from build123d import *

# Parameters (mm, degrees)
SKETCH_1_W          = 290
SKETCH_1_H          = 50
EXTRUDE_1_DEPTH     = 5
SKETCH_3_W          = 20
SKETCH_3_H          = 50
CUT_EXTRUDE_1_DEPTH = 10
SKETCH_4_W          = 150
SKETCH_4_H          = 5
EXTRUDE_2_DEPTH     = 10
SKETCH_5_R          = 2.75
CUT_EXTRUDE_4_DEPTH = 130.903810568
CUT_EXTRUDE_5_DEPTH = 10


with BuildPart() as part:
    # 스케치1 → 보스-돌출1 (new body)
    with BuildSketch(Plane.XY):
        Rectangle(SKETCH_1_W, SKETCH_1_H)
    extrude(amount=EXTRUDE_1_DEPTH)

    # 스케치3 → 컷-돌출1 (cut)
    with BuildSketch(Plane.XY.offset(5)):
        with Locations((-135, 0)):
            Rectangle(SKETCH_3_W, SKETCH_3_H)
    cut_extrude_1 = extrude(amount=-CUT_EXTRUDE_1_DEPTH, mode=Mode.SUBTRACT)

    # 대칭 복사1: 컷-돌출1 across plane
    add(cut_extrude_1.mirror(Plane(origin=(0, 0, 0), x_dir=(0, 0, 1), z_dir=(1, 0, 0))), mode=Mode.SUBTRACT)

    # 스케치4 → 보스-돌출2 (add)
    with BuildSketch(Plane(origin=(0, 25, 0), x_dir=(1, 0, 0), z_dir=(0, 1, 0))):
        with Locations((0, -2.5)):
            Rectangle(SKETCH_4_W, SKETCH_4_H)
    extrude(amount=EXTRUDE_2_DEPTH)

    # 스케치5 → 컷-돌출4 (cut, through all)
    with BuildSketch(Plane.XY.offset(5)):
        with Locations((-84, 15)):
            Circle(SKETCH_5_R)
        with Locations((-116, 15)):
            Circle(SKETCH_5_R)
        with Locations(Location((116, 15, 0), (0, 0, 180))):
            Circle(SKETCH_5_R)
        with Locations(Location((84, 15, 0), (0, 0, 180))):
            Circle(SKETCH_5_R)
    extrude(amount=-CUT_EXTRUDE_4_DEPTH, mode=Mode.SUBTRACT)

    # 스케치6 → 컷-돌출5 (cut)
    with BuildSketch(Plane.XY.offset(5)):
        with BuildLine():
            Line((59.99900565, 22.696938457), (59.99900565, -6.696938457))
            ThreePointArc((59.99900565, -6.696938457), (44.99900565, -13), (29.99900565, -6.696938457))
            Line((29.99900565, -6.696938457), (29.99900565, 22.696938457))
            ThreePointArc((29.99900565, 22.696938457), (44.99900565, 29), (59.99900565, 22.696938457))
        make_face()
    cut_extrude_5 = extrude(amount=-CUT_EXTRUDE_5_DEPTH, mode=Mode.SUBTRACT)

    # 대칭 복사2: 컷-돌출5 across plane
    add(cut_extrude_5.mirror(Plane.ZY), mode=Mode.SUBTRACT)


solid = part.part
Work out the finished part from the listing and answer in its coordinate system (mm). A direction names the side the tool comes from. Give positions to 0.01 mm unless a question says otherwise; leave off trailing zeros. Loops run counter-clockwise (first coordinate to the right, second up) from the corner with the lowest first, then second, coordinate; pieces in that order, holes last. Notation, with made-up numbers: (13, 76.5) - (63, 76.5) arc R33 cw to (63, 115.5) - close; hole circle Ø5 at (72, 9). An arc over 180 degrees is marked (long way). Answer in a Markdown table with one row per item.
(1) Section C-C (y = 15) is taken. Give the vertices of the cut face in (x, z), and give its area (3 significant figures).
Results list:
| item | result |
|---|---|
| outline | (-125, 0) - (-118.75, 0) - (-118.75, 5) - (-125, 5) - close; (-113.25, 0) - (-86.75, 0) - (-86.75, 5) - (-113.25, 5) - close; (-81.25, 0) - (-60, 0) - (-60, 5) - (-81.25, 5) - close; (-30, 0) - (30, 0) - (30, 5) - (-30, 5) - close; (60, 0) - (81.25, 0) - (81.25, 5) - (60, 5) - close; (86.75, 0) - (113.25, 0) - (113.25, 5) - (86.75, 5) - close; (118.75, 0) - (125, 0) - (125, 5) - (118.75, 5) - close |
| area | 840 mm² |
(2) Section A-A (z = 2.85) is taken. Give the vertices of the cut face in (x, y), and give its area (3 significant figures).
Results list:
| item | result |
|---|---|
| outline | (-125, -25) - (125, -25) - (125, 25) - (75, 25) - (75, 35) - (-75, 35) - (-75, 25) - (-125, 25) - close; hole circle Ø5.5 at (-116, 15); hole circle Ø5.5 at (-84, 15); hole (-60, -6.7) arc R21 ccw to (-30, -6.7) - (-30, 22.7) arc R21 ccw to (-60, 22.7) - close; hole (30, -6.7) arc R21 ccw to (60, -6.7) - (60, 22.7) arc R21 ccw to (30, 22.7) - close; hole circle Ø5.5 at (84, 15); hole circle Ø5.5 at (116, 15) |
| area | 11,600 mm² |
(3) A tool of negligible diameter and unlimited length cuts with its end or side. For faces 1 (the face through (-100, 25, 2)), 2 (the face through (-29.999, 8, 3)), 3 (the face through (-1, 35, 2)), 4 (the face through (100, 25, 2)), from which of +Z, -Z, +X, -X, +Y, -Y can it reach the whole face along a straight path? Write none if from no direction.
Results list:
| item | result |
|---|---|
| face 1 | +Z, -Z, -X, +Y |
| face 2 | +Z, -Z |
| face 3 | +Z, -Z, +X, -X, +Y |
| face 4 | +Z, -Z, +X, +Y |
(4) Consider L1, parallel to X at y = -5.5, z = 3.4; L2, parallel to Y at x = 84, z = 3.35; L3, parallel to Y at x = -54, z = 4.25. Determine where each line is inside the solid, lowest interval first. Write a range as [from, to].
Results list:
| item | result |
|---|---|
| L1 | x = [-125, -60], [-30, 30], [60, 125] |
| L2 | y = [-25, 12.25], [17.75, 25] |
| L3 | y = [-25, -10.97], [26.97, 35] |
(5) Section D-D (x = 53.5) is taken. Give the vertices of the cut face in (y, z), and give its area (3 significant figures).
Results list:
| item | result |
|---|---|
| outline | (-25, 0) - (-11.2, 0) - (-11.2, 5) - (-25, 5) - close; (27.2, 0) - (35, 0) - (35, 5) - (27.2, 5) - close |
| area | 108 mm² |
(6) Section B-B (x = -84) is taken. Give the vertices of the cut face in (y, z), and give its area (4 significant figures).
Results list:
| item | result |
|---|---|
| outline | (-25, 0) - (12.25, 0) - (12.25, 5) - (-25, 5) - close; (17.75, 0) - (25, 0) - (25, 5) - (17.75, 5) - close |
| area | 222.5 mm² |
(7) Flat-ended cylindrical pins translate along their axes: pin 1 Ø2.5 at (y, z) = (30.5, 3.5) entering from -X; pin 2 Ø1.5 at (y, z) = (32, 3) entering from +X; pin 3 Ø4.5 at (x, y) = (84, 15) entering from -Z; pin 4 Ø1.5 at (x, z) = (-92.5, 3.5) entering from +Y. Find the tip coordinate at first contact, or state that the pin passes through.
Results list:
| item | result |
|---|---|
| pin 1 | stops at x = -75 |
| pin 2 | stops at x = 75 |
| pin 3 | passes through |
| pin 4 | stops at y = 25 |
(8) For a pull along X with two mould halves and no side action, classify faces 5 (the face through (-125, 0, 3)), 6 (the face through (-45, 29, 3)), 7 (the face through (-2, -1, 0)) as pulls with the +X half, pulls with the -X half, needs draft (parallel to the pull), parting line crosses it, or undercut.
Results list:
| item | result |
|---|---|
| face 5 | pulls with the -X half |
| face 6 | undercut |
| face 7 | needs draft |
